The model under review builds one solid part; all positions refer to its coordinate system, in mm. Round coordinates to 2 decimals unless told otherwise and drop trailing zeros. Write each loop counter-clockwise with the first axis right and the second up, starting at its lowest first coordinate (ties: lowest second). Pieces come first, ordered by that corner, then holes.
Item 1: Add section B-B (x = 18.3). Give the boundary of the cut face in (y, z), plus the area to 3 significant figures.
Item 2: Add section D-D (y = -2.1). State how many separate pieces and enclosed holes the cut face has, plus the area to 3 significant figures.
Item 3: Draft analysis for pull direction X (two halves, no side actions). For faces 1 (the face through (23.6, -1.52, -19.24)), 2 (the face through (-24.199, -3.715, 0.239)), 3 (the face through (23, -2, 0)), 4 (the face through (0, -4, -17)), state which applies: +X half, -X half, draft (parallel to the pull), parting line (faces both ways), or undercut.
Item 4: Add section A-A (z = -13.85). Give the boundary of the cut face in (x, y), plus the area to 3 significant figures.
Item 5: To check wall thickness, follow L1, parallel to Z at x = 0, y = -2; L2, parallel to Z at x = -18.3, y = -1.65; L3, parallel to X at y = -1.95, z = 12.5. State the ranges of each line that lie inside material, in increasing order.
Item 6: Add section C-C (x = -8.5). Give the boundary of the cut face in (y, z), plus the area to 3 significant figures.
```python
from build123d import *

# Parameters (mm, degrees)
F0_W     = 49
F0_H     = 40.2
F0_R     = 0.5
F0_R_2   = 1
F0_W_2   = 32.2
F0_H_2   = 32.2
F1_DEPTH = 4
F2_R     = 3
F3_R     = 1


with BuildPart() as f1:
    # F0 (on Front) → F1 (new body)
    with BuildSketch(Plane.XZ):
        Rectangle(F0_W, F0_H)
        with Locations((-22.5, -18.1)):
            Circle(F0_R, mode=Mode.SUBTRACT)
        with Locations((-18.3, -13.85)):
            Circle(F0_R_2, mode=Mode.SUBTRACT)
        with Locations((0, -18.1)):
            Circle(F0_R, mode=Mode.SUBTRACT)
        with Locations((22.5, -18.1)):
            Circle(F0_R, mode=Mode.SUBTRACT)
        with Locations((18.3, -13.85)):
            Circle(F0_R_2, mode=Mode.SUBTRACT)
        with Locations((-22.5, 0)):
            Circle(F0_R, mode=Mode.SUBTRACT)
        Rectangle(F0_W_2, F0_H_2, mode=Mode.SUBTRACT)
        with Locations((-18.3, 13.85)):
            Circle(F0_R_2, mode=Mode.SUBTRACT)
        with Locations((-22.5, 18.1)):
            Circle(F0_R, mode=Mode.SUBTRACT)
        with Locations((0, 18.1)):
            Circle(F0_R, mode=Mode.SUBTRACT)
        with Locations((22.5, 0)):
            Circle(F0_R, mode=Mode.SUBTRACT)
        with Locations((18.3, 13.85)):
            Circle(F0_R_2, mode=Mode.SUBTRACT)
        with Locations((22.5, 18.1)):
            Circle(F0_R, mode=Mode.SUBTRACT)
    extrude(amount=F1_DEPTH)

    # F2
    f2_edges = [f1.edges().sort_by_distance(p)[0] for p in [
        (-24.5, -2, -20.1),
        (24.5, -2, -20.1),
        (24.5, -2, 20.1),
        (-24.5, -2, 20.1),
    ]]
    fillet(f2_edges, radius=F2_R)

    # F3
    f3_edges = [f1.edges().sort_by_distance(p)[0] for p in [
        (0, -4, 20.1),
    ]]
    fillet(f3_edges, radius=F3_R)


solid = f1.part
```
Numbers:
1. outline: (-4, -19.1) arc R1 ccw to (-3, -20.1) - (0, -20.1) - (0, -14.85) - (-4, -14.85) - close; (-4, -12.85) - (0, -12.85) - (0, 12.85) - (-4, 12.85) - close; (-4, 14.85) - (0, 14.85) - (0, 20.1) - (-3, 20.1) arc R1 ccw to (-4, 19.1) - close
1. area: 144 mm2
2. separate pieces: 1
2. enclosed holes: 13
2. area: 906 mm2
3. face 1: +X half
3. face 2: -X half
3. face 3: undercut
3. face 4: draft
4. outline: (-24.5, -3) arc R1 ccw to (-23.5, -4) - (-19.3, -4) - (-19.3, 0) - (-24.5, 0) - close; (-17.3, -4) - (-16.1, -4) - (-16.1, 0) - (-17.3, 0) - close; (16.1, -4) - (17.3, -4) - (17.3, 0) - (16.1, 0) - close; (19.3, -4) - (23.5, -4) arc R1 ccw to (24.5, -3) - (24.5, 0) - (19.3, 0) - close
4. area: 50.8 mm2
5. L1: z = -20.1 to -18.6, -17.6 to -16.1, 16.1 to 17.6, 18.6 to 20.1
5. L2: z = -20.1 to -14.85, -12.85 to 12.85, 14.85 to 20.1
5. L3: x = -24.5 to -16.1, 16.1 to 24.5
6. outline: (-4, -19.1) arc R1 ccw to (-3, -20.1) - (0, -20.1) - (0, -16.1) - (-4, -16.1) - close; (-4, 16.1) - (0, 16.1) - (0, 20.1) - (-3, 20.1) arc R1 ccw to (-4, 19.1) - close
6. area: 31.6 mm2
